from build123d import *

# Parameters (mm, degrees)
ESQUISSE1_W             = 25
ESQUISSE1_H             = 26
ESQUISSE1_R             = 1.5
BOSS_EXTRU_1_DEPTH      = 2
BOSS_EXTRU_2_DEPTH      = 26
BOSS_EXTRU_3_DEPTH      = 2
ESQUISSE7_R             = 1.5
ENL_V_MAT_EXTRU_1_DEPTH = 3
ESQUISSE6_R             = 5
ENL_V_MAT_EXTRU_2_DEPTH = 28
ESQUISSE8_R             = 1.25
ENL_V_MAT_EXTRU_3_DEPTH = 28


with BuildPart() as part:
    # Esquisse1 → Boss.-Extru.1 (new body)
    with BuildSketch(Plane.XY):
        Rectangle(ESQUISSE1_W, ESQUISSE1_H)
        with Locations((-6.25, 6.5)):
            Circle(ESQUISSE1_R, mode=Mode.SUBTRACT)
        with Locations((6.25, 6.5)):
            Circle(ESQUISSE1_R, mode=Mode.SUBTRACT)
        with Locations((6.25, -6.5)):
            Circle(ESQUISSE1_R, mode=Mode.SUBTRACT)
        with Locations((-6.25, -6.5)):
            Circle(ESQUISSE1_R, mode=Mode.SUBTRACT)
    extrude(amount=BOSS_EXTRU_1_DEPTH)

    # Esquisse2 → Boss.-Extru.2 (add)
    with BuildSketch(Plane(origin=(0, 13, 0), x_dir=(1, 0, 0), z_dir=(0, 1, 0))):
        with BuildLine():
            Line((-12.5, -2), (12.5, -2))
            Line((12.5, -2), (12.5, 0))
            Line((12.5, 0), (-12.5, 0))
            Line((-12.5, 0), (-12.5, 14.15))
            Line((-12.5, 14.15), (-14.5, 14.15))
            Line((-14.5, 14.15), (-14.5, 0))
            ThreePointArc((-14.5, 0), (-13.914213562, -1.414213562), (-12.5, -2))
        make_face()
    extrude(amount=-BOSS_EXTRU_2_DEPTH)

    # Esquisse5 → Boss.-Extru.3 (add)
    with BuildSketch(Plane.ZY.offset(14.5)):
        with BuildLine():
            Line((-14.15, -13), (-14.15, 13))
            ThreePointArc((-14.15, 13), (-27.15, 0), (-14.15, -13))
        make_face()
    extrude(amount=-BOSS_EXTRU_3_DEPTH)

    # Esquisse7 → Enlèv. mat.-Extru.1 (cut, through all)
    with BuildSketch(Plane(origin=(0, 0, 0), x_dir=(-1, 0, 0), z_dir=(0, 0, -1))):
        with Locations((-6.25, -6.5)):
            Circle(ESQUISSE7_R)
        with Locations((6.25, -6.5)):
            Circle(ESQUISSE7_R)
        with Locations((6.25, 6.5)):
            Circle(ESQUISSE7_R)
        with Locations((-6.25, 6.5)):
            Circle(ESQUISSE7_R)
    extrude(amount=-ENL_V_MAT_EXTRU_1_DEPTH, mode=Mode.SUBTRACT)

    # Esquisse6 → Enlèv. mat.-Extru.2 (cut, through all)
    with BuildSketch(Plane.ZY.offset(14.5)):
        with Locations((-14.15, 0)):
            Circle(ESQUISSE6_R)
    extrude(amount=-ENL_V_MAT_EXTRU_2_DEPTH, mode=Mode.SUBTRACT)

    # Esquisse8 → Enlèv. mat.-Extru.3 (cut, through all)
    with BuildSketch(Plane.ZY.offset(14.5)):
        with Locations((-14.15, 8.5)):
            Circle(ESQUISSE8_R)
        with Locations((-14.15, -8.5)):
            Circle(ESQUISSE8_R)
    extrude(amount=-ENL_V_MAT_EXTRU_3_DEPTH, mode=Mode.SUBTRACT)


solid = part.part
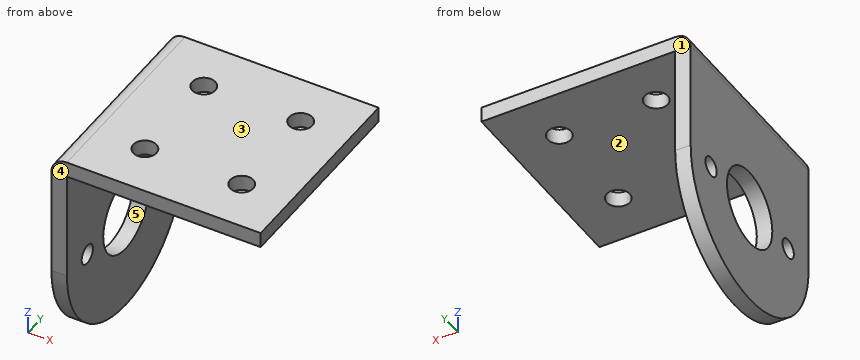
CAD build for the part. Positions are in the model's coordinates, mm. Face numbers are marked on the shaded views. A direction names the side the tool comes from. Round coordinates to 2 decimals unless told otherwise and drop trailing zeros. Write each loop counter-clockwise with the first axis right and the second up, starting at its lowest first coordinate (ties: lowest second). Pieces come first, ordered by that corner, then holes. Notation, with made-up numbers: (40, -17) -> (74, -17) arc R28 ccw to (74, 8) -> close; hole circle Ø9 at (17.25, 58). An arc over 180 degrees is marked (long way). Answer as a JSON object with one key per item and string values.
(1) Probe probe 1 along Y at (x, z) = (-14.1, -14.15); probe 2 along Y at (x, z) = (6.25, 0.9); probe 3 along X at (y, z) = (0.5, -8.25). List the from-to ranges inside material, lowest first. Write a range as [from, to].
Reported:
{"probe 1": "y = [-13, -9.75], [-7.25, -5], [5, 7.25], [9.75, 13]", "probe 2": "y = [-13, -8], [-5, 5], [8, 13]", "probe 3": "x = [-14.5, -12.5]"}
(2) Pin check, flat tips, straight feed: P1, Ø7.5, axis at x = 3.5, y = 3, coming from the -Z side; P2, Ø8, axis at y = -4, z = -8, coming from the +X side. Stop position of each tip, or through.
Reported:
{"P1": "stops at z = 0", "P2": "stops at x = -12.5"}
(3) Two-plate mould, pull along Y, no slides. Class the marked faces 3, 4 and 5: +Y half, -Y half, draft (parallel to the pull), parting line (faces both ways), or undercut.
Reported:
{"face 3": "draft", "face 4": "-Y half", "face 5": "undercut"}
(4) Band-saw the part on D-D, the plane z = -16.5. List the corners of the cut face in (x, y), then the cut area to 3 significant figures.
Reported:
{"outline": "(-14.5, -12.79) -> (-12.5, -12.79) -> (-12.5, -4.41) -> (-14.5, -4.41) -> close; (-14.5, 4.41) -> (-12.5, 4.41) -> (-12.5, 12.79) -> (-14.5, 12.79) -> close", "area": "33.5 mm^2"}
(5) Band-saw the part on A-A, the plane x = 6.25. List the corners of the cut face in (y, z), then the cut area to 3 significant figures.
Reported:
{"outline": "(-13, 0) -> (-8, 0) -> (-8, 2) -> (-13, 2) -> close; (-5, 0) -> (5, 0) -> (5, 2) -> (-5, 2) -> close; (8, 0) -> (13, 0) -> (13, 2) -> (8, 2) -> close", "area": "40.0 mm^2"}
(6) Band-saw the part on B-B, the plane y = -6.5. List the corners of the cut face in (x, z), then the cut area to 3 significant figures.
Reported:
{"outline": "(-14.5, -25.41) -> (-12.5, -25.41) -> (-12.5, 0) -> (-7.75, 0) -> (-7.75, 2) -> (-12.5, 2) arc R2 ccw to (-14.5, 0) -> close; (-4.75, 0) -> (4.75, 0) -> (4.75, 2) -> (-4.75, 2) -> close; (7.75, 0) -> (12.5, 0) -> (12.5, 2) -> (7.75, 2) -> close", "area": "92.0 mm^2"}
(7) Which spindle directions (+Z, -Z, +X, -X, +Y, -Y) get a long thin tool onto all of the face, cutting with end or side? Do the marked faces 1 and 2. Say none if no direction does.
Reported:
{"face 1": "+Z, -Z, +X, -X, +Y", "face 2": "-Z, +X, +Y, -Y"}
(8) Band-saw the part on C-C, the plane z = -13.5. List the corners of the cut face in (x, y).
Reported:
{"outline": "(-14.5, -13) -> (-12.5, -13) -> (-12.5, -9.57) -> (-14.5, -9.57) -> close; (-14.5, -7.43) -> (-12.5, -7.43) -> (-12.5, -4.96) -> (-14.5, -4.96) -> close; (-14.5, 4.96) -> (-12.5, 4.96) -> (-12.5, 7.43) -> (-14.5, 7.43) -> close; (-14.5, 9.57) -> (-12.5, 9.57) -> (-12.5, 13) -> (-14.5, 13) -> close"}
